Verification items for the finished model (mm, model axes). A direction names the side the tool comes from. Coordinates: 2 decimals unless noted, no trailing zeros. Order: outer loops, then holes, each group sorted by start corner. A loop starts at its lowest first (then second) coordinate and runs counter-clockwise, first axis right, second up.
Q1. Cross-section at C-C, the plane z = 12.25. Record the boundary of the cut face in (x, y), and give its area (3 significant figures).
Q2. Set-up check for faces 1 (the flat face through (-5, 25.75, 2)), 2 (the flat face through (-36.35, 27.63, 6)), 3 (the flat face through (24, -30.968, 9)), 4 (the flat face through (43, 25.77, 2)), 5 (the flat face through (-60, -32, 3)): record each of +Z, -Z, +X, -X, +Y, -Y from which the full face is reachable in a straight line by a thin tool's end or side.
Q3. Cross-section at A-A, the plane x = 43. Record the boundary of the cut face in (y, z).
Q4. Depth check by flat-ended pin: P1, Ø12, axis at x = -1.5, y = 4, coming from the +Z side; P2, Ø1.6, axis at x = 19.5, z = 1, coming from the +Y side; P3, Ø2.5, axis at x = 24, z = 11, coming from the -Y side. Enter the tip coordinate at first touch or a pass-through.
Q5. Draft check along X on faces 6 (the flat face through (59.706, -6, 1)), 7 (the flat face through (-58, -30, 3)), 8 (the flat face through (1, 0, 0)). Enter one of: pulls with the +X half, pulls with the -X half, needs draft (parallel to the pull), parting line crosses it, or undercut.
Q6. Thickness scan on line 1 (Y direction, x = 24.5, z = 11); line 2 (Y direction, x = 54.5, z = 1.25); line 3 (Y direction, x = 31.5, z = 2.5). Record the ranges inside material, lowest first.
Q7. Cross-section at B-B, the plane y = -18.65. Record the boundary of the cut face in (x, z), and give its area (3 significant figures).
Q8. Cross-section at D-D, the plane y = 23.5. Record the boundary of the cut face in (x, z), and give its area (3 significant figures).
from build123d import *

# Parameters (mm, degrees)
SKETCH1_R           = 1.35
BOSS_EXTRUDE1_DEPTH = 3
SKETCH2_W           = 32.539262004
SKETCH2_H           = 47.2
CUT_EXTRUDE1_DEPTH  = 1.5
CUT_EXTRUDE2_DEPTH  = 1
SKETCH4_W           = 39.18
SKETCH4_H           = 5.04
CUT_EXTRUDE3_DEPTH  = 3
BOSS_EXTRUDE3_START = -1
SKETCH5_W           = 3.213705867
SKETCH5_H           = 5.217642876
BOSS_EXTRUDE3_DEPTH = 15
SKETCH6_R           = 2.35
BOSS_EXTRUDE4_DEPTH = 6
SKETCH7_R           = 1.35
CUT_EXTRUDE4_DEPTH  = 3
SKETCH8_R           = 1.799931462
BOSS_EXTRUDE5_DEPTH = 8
SKETCH9_R           = 1
CUT_EXTRUDE5_DEPTH  = 11
CUT_EXTRUDE6_DEPTH  = 3
SKETCH11_W          = 50.12494376
SKETCH11_H          = 8
CUT_EXTRUDE7_DEPTH  = 3
SKETCH12_W          = 2.262523605
SKETCH12_H          = 18.069154429
CUT_EXTRUDE8_DEPTH  = 1.75
SKETCH13_R          = 1.75
CUT_EXTRUDE9_DEPTH  = 3


with BuildPart() as part:
    # Sketch1 → Boss-Extrude1 (new body)
    with BuildSketch(Plane.XY):
        Polygon((59.70625, -28.75), (59.70625, -32.25), (59.20625, -32.75), (51.936987996, -32.75), (51.436987996, -32.25), (51.436987996, -30.75), (40.496987996, -30.75), (40.496987996, -32.25), (39.996987996, -32.75), (35.916987996, -32.75), (35.416987996, -32.25), (35.416987996, -30.75), (26.916987996, -30.75), (26.916987996, -32.25), (26.416987996, -32.75), (22.416987996, -32.75), (21.916987996, -32.25), (21.916987996, -30.75), (13.416987996, -30.75), (13.416987996, -32.25), (12.916987996, -32.75), (8.166987996, -32.75), (7.666987996, -32.25), (7.666987996, -30.75), (-7.666987996, -30.75), (-7.666987996, -32.25), (-8.166987996, -32.75), (-12.916987996, -32.75), (-13.416987996, -32.25), (-13.416987996, -30.75), (-21.916987996, -30.75), (-21.916987996, -32.25), (-22.416987996, -32.75), (-26.416987996, -32.75), (-26.916987996, -32.25), (-26.916987996, -30.75), (-35.416987996, -30.75), (-35.416987996, -32.25), (-35.916987996, -32.75), (-39.996987996, -32.75), (-40.496987996, -32.25), (-40.496987996, -30.75), (-51.436987996, -30.75), (-51.436987996, -32.25), (-51.936987996, -32.75), (-59.663932929, -32.75), (-60.163932929, -32.25), (-60.163932929, 32.25), (-59.663932929, 32.75), (-51.936987996, 32.75), (-51.436987996, 32.25), (-51.436987996, 30.75), (-40.496987996, 30.75), (-40.496987996, 32.25), (-39.996987996, 32.75), (-35.916987996, 32.75), (-35.416987996, 32.25), (-35.416987996, 30.75), (7.666987996, 30.75), (7.666987996, 32.25), (8.166987996, 32.75), (12.916987996, 32.75), (13.416987996, 32.25), (13.416987996, 30.75), (21.916987996, 30.75), (21.916987996, 32.25), (22.416987996, 32.75), (26.416987996, 32.75), (26.916987996, 32.25), (26.916987996, 30.75), (35.416987996, 30.75), (35.416987996, 32.25), (35.916987996, 32.75), (39.996987996, 32.75), (40.496987996, 32.25), (40.496987996, 30.75), (51.436987996, 30.75), (51.436987996, 32.25), (51.936987996, 32.75), (59.20625, 32.75), (59.70625, 32.25), (59.70625, 28.75), align=None)
        with Locations((10.545756529, 30.750001775)):
            Circle(SKETCH1_R, mode=Mode.SUBTRACT)
        with Locations((55.575387531, 30.750001775)):
            Circle(SKETCH1_R, mode=Mode.SUBTRACT)
        with Locations((55.571618998, -30.75)):
            Circle(SKETCH1_R, mode=Mode.SUBTRACT)
        with Locations((10.541987996, -30.75)):
            Circle(SKETCH1_R, mode=Mode.SUBTRACT)
        with Locations((-24.416987996, -30.75)):
            Circle(SKETCH1_R, mode=Mode.SUBTRACT)
    extrude(amount=BOSS_EXTRUDE1_DEPTH)

    # Sketch2 → Cut-Extrude1 (cut)
    with BuildSketch(Plane.XY.offset(3)):
        with Locations((43.436618998, -2.1)):
            Rectangle(SKETCH2_W, SKETCH2_H)
    extrude(amount=-CUT_EXTRUDE1_DEPTH, mode=Mode.SUBTRACT)

    # Sketch3 → Cut-Extrude2 (cut)
    with BuildSketch(Plane.XY.offset(3)):
        with BuildLine():
            Line((7.666987996, 28.75), (8.309690139, 28.75))
            ThreePointArc((8.309690139, 28.75), (10.545756529, 27.750001775), (12.781822919, 28.75))
            Line((12.781822919, 28.75), (53.339321141, 28.75))
            ThreePointArc((53.339321141, 28.75), (55.575387531, 27.750001775), (57.811453921, 28.75))
            Line((57.811453921, 28.75), (59.70625, 28.75))
            Line((59.70625, 28.75), (59.70625, 32.75))
            Line((59.70625, 32.75), (7.666987996, 32.75))
            Line((7.666987996, 32.75), (7.666987996, 28.75))
        make_face()
        with BuildLine():
            Line((-31.069252348, -28.75), (-26.653055973, -28.75))
            ThreePointArc((-26.653055973, -28.75), (-24.416987996, -27.75), (-22.180920018, -28.75))
            Line((-22.180920018, -28.75), (8.305920018, -28.75))
            ThreePointArc((8.305920018, -28.75), (10.541987996, -27.75), (12.778055973, -28.75))
            Line((12.778055973, -28.75), (53.33555102, -28.75))
            ThreePointArc((53.33555102, -28.75), (55.571618998, -27.75), (57.807686975, -28.75))
            Line((57.807686975, -28.75), (59.70625, -28.75))
            Line((59.70625, -28.75), (59.70625, -32.75))
            Line((59.70625, -32.75), (-22.180920018, -32.75))
            ThreePointArc((-22.180920018, -32.75), (-24.416987996, -33.75), (-26.653055973, -32.75))
            Line((-26.653055973, -32.75), (-31.069252348, -32.75))
            Line((-31.069252348, -32.75), (-31.069252348, -28.75))
        make_face()
    extrude(amount=-CUT_EXTRUDE2_DEPTH, mode=Mode.SUBTRACT)

    # Sketch4 → Cut-Extrude3 (cut)
    with BuildSketch(Plane.XY.offset(3)):
        with Locations((47.236987996, 23.25)):
            Rectangle(SKETCH4_W, SKETCH4_H)
    extrude(amount=-CUT_EXTRUDE3_DEPTH, mode=Mode.SUBTRACT)

    # Sketch5 → Boss-Extrude3 (add)
    with BuildSketch(Plane.XY.offset(3).offset(BOSS_EXTRUDE3_START)):
        with Locations((24.416987996, -28.358821438)):
            Rectangle(SKETCH5_W, SKETCH5_H)
        with Locations((24.416987996, 28.258821438)):
            Rectangle(SKETCH5_W, SKETCH5_H)
    extrude(amount=BOSS_EXTRUDE3_DEPTH)

    # Sketch6 → Boss-Extrude4 (add)
    with BuildSketch(Plane(origin=(0, 0, 0), x_dir=(-1, 0, 0), z_dir=(0, 0, -1))):
        with Locations((57.813932929, -30.4)):
            Circle(SKETCH6_R)
        with Locations((34.814808698, -30.4)):
            Circle(SKETCH6_R)
        with Locations((34.814808698, 27.597791538)):
            Circle(SKETCH6_R)
        with Locations((57.813932929, 27.597791538)):
            Circle(SKETCH6_R)
    extrude(amount=-BOSS_EXTRUDE4_DEPTH)

    # Sketch7 → Cut-Extrude4 (cut)
    with BuildSketch(Plane.XY.offset(6)):
        with Locations((-57.813932929, 27.597791538)):
            Circle(SKETCH7_R)
        with Locations((-34.814808698, 27.597791538)):
            Circle(SKETCH7_R)
        with Locations((-34.814808698, -30.4)):
            Circle(SKETCH7_R)
        with Locations((-57.813932929, -30.4)):
            Circle(SKETCH7_R)
    extrude(amount=-CUT_EXTRUDE4_DEPTH, mode=Mode.SUBTRACT)

    # Sketch8 → Boss-Extrude5 (add)
    with BuildSketch(Plane.XY.offset(3)):
        with Locations(Location((-34.249007268, -1.671088179, 0), (0, 0, 180))):
            Circle(SKETCH8_R)
        with Locations(Location((-21.949943943, -1.778420479, 0), (0, 0, 180))):
            Circle(SKETCH8_R)
        with Locations(Location((-22.124474985, -22.777697016, 0), (0, 0, 180))):
            Circle(SKETCH8_R)
        with Locations(Location((-34.432264513, -22.670288564, 0), (0, 0, 180))):
            Circle(SKETCH8_R)
    extrude(amount=BOSS_EXTRUDE5_DEPTH)

    # Sketch9 → Cut-Extrude5 (cut)
    with BuildSketch(Plane.XY.offset(11)):
        with Locations((-34.432264513, -22.670288564)):
            Circle(SKETCH9_R)
        with Locations((-22.133201188, -22.777620863)):
            Circle(SKETCH9_R)
        with Locations((-34.249007268, -1.671088179)):
            Circle(SKETCH9_R)
        with Locations((-21.949943943, -1.778420479)):
            Circle(SKETCH9_R)
    extrude(amount=-CUT_EXTRUDE5_DEPTH, mode=Mode.SUBTRACT)

    # Sketch10 → Cut-Extrude6 (cut)
    with BuildSketch(Plane.XY.offset(3)):
        with BuildLine():
            Line((-2.078617038, -24.770288564), (-2.068617038, -24.770288564))
            ThreePointArc((-2.068617038, -24.770288564), (-1.361510257, -24.477395345), (-1.068617038, -23.770288564))
            Line((-1.068617038, -23.770288564), (-1.068617038, -0.570288564))
            ThreePointArc((-1.068617038, -0.570288564), (-1.361510257, 0.136818218), (-2.068617038, 0.429711436))
            Line((-2.068617038, 0.429711436), (-2.078617038, 0.429711436))
            ThreePointArc((-2.078617038, 0.429711436), (-2.785723819, 0.136818218), (-3.078617038, -0.570288564))
            Line((-3.078617038, -0.570288564), (-3.078617038, -23.770288564))
            ThreePointArc((-3.078617038, -23.770288564), (-2.785723819, -24.477395345), (-2.078617038, -24.770288564))
        make_face()
    extrude(amount=-CUT_EXTRUDE6_DEPTH, mode=Mode.SUBTRACT)

    # Sketch11 → Cut-Extrude7 (cut)
    with BuildSketch(Plane.XY.offset(3)):
        with Locations((-4.252336818, 21.750001775)):
            Rectangle(SKETCH11_W, SKETCH11_H)
    extrude(amount=-CUT_EXTRUDE7_DEPTH, mode=Mode.SUBTRACT)

    # Sketch12 → Cut-Extrude8 (cut)
    with BuildSketch(Plane.XY.offset(11)):
        with Locations((-34.432264514, -12.23571135)):
            Rectangle(SKETCH12_W, SKETCH12_H)
    extrude(amount=-CUT_EXTRUDE8_DEPTH, mode=Mode.SUBTRACT)

    # Sketch13 → Cut-Extrude9 (cut)
    with BuildSketch(Plane.XY.offset(3)):
        with Locations((19.092279678, -18.65)):
            Circle(SKETCH13_R)
        with Locations((2.066987996, -18.65)):
            Circle(SKETCH13_R)
    extrude(amount=-CUT_EXTRUDE9_DEPTH, mode=Mode.SUBTRACT)


solid = part.part
Check values:
1. outline: (22.81, -30.97) - (26.02, -30.97) - (26.02, -25.75) - (22.81, -25.75) - close; (22.81, 25.65) - (26.02, 25.65) - (26.02, 30.87) - (22.81, 30.87) - close
1. area: 33.5 mm2
2. face 1: +Z, -Z
2. face 2: +Z, -X, +Y
2. face 3: +Z, +X, -Y
2. face 4: +Z, -Z, +X
2. face 5: +Z, -X, -Y
3. outline: (-30.75, 0) - (20.73, 0) - (20.73, 1.5) - (-25.7, 1.5) - (-25.7, 3) - (-28.75, 3) - (-28.75, 2) - (-30.75, 2) - close; (25.77, 0) - (30.75, 0) - (30.75, 2) - (28.75, 2) - (28.75, 3) - (25.77, 3) - close
4. P1: stops at z = 3
4. P2: stops at y = 30.75
4. P3: stops at y = -30.97
5. face 6: pulls with the +X half
5. face 7: undercut
5. face 8: needs draft
6. line 1: y = -30.97 to -25.75, 25.65 to 30.87
6. line 2: y = -32.75 to -31.57, -29.93 to 20.73, 25.77 to 29.93, 31.57 to 32.75
6. line 3: y = -28.75 to -25.7, 25.77 to 28.75
7. outline: (-60.16, 0) - (-3.08, 0) - (-3.08, 3) - (-60.16, 3) - close; (-1.07, 0) - (0.32, 0) - (0.32, 3) - (-1.07, 3) - close; (3.82, 0) - (17.34, 0) - (17.34, 3) - (3.82, 3) - close; (20.84, 0) - (59.71, 0) - (59.71, 1.5) - (27.17, 1.5) - (27.17, 3) - (20.84, 3) - close
7. area: 284 mm2
8. outline: (-60.16, 0) - (-29.31, 0) - (-29.31, 3) - (-60.16, 3) - close; (20.81, 0) - (27.65, 0) - (27.65, 3) - (20.81, 3) - close
8. area: 113 mm2
